Autodesk Inventor part; units mm, degrees
ref_plane "YZ Plane" through (0, 0, 0) normal (1, 0, 0) x (0, 1, 0)
ref_plane "XZ Plane" through (0, 0, 0) normal (0, 1, 0) x (-1, 0, 0)
ref_plane "XY Plane" through (0, 0, 0) normal (0, 0, 1) x (1, 0, 0)
sketch "Sketch1" plane through (0, 0, 0) normal (0, 1, 0) x (-1, 0, 0)
  line L0 (-19.3459, 17.7433) -> (-1.3259, 17.7433)
  line L1 (-1.3259, 0.9433) -> (-19.3459, 0.9433)
  line L2 (-19.3459, 14.5433) -> (-24.3459, 14.5433)
  line L3 (-24.3459, 14.5433) -> (-24.3459, 12.5433)
  line L4 (-24.3459, 12.5433) -> (-19.3459, 12.5433)
  line L5 (-19.3459, 17.7433) -> (-19.3459, 14.5433)
  line L6 (-19.3459, 12.5433) -> (-19.3459, 0.9433)
  line L7 (-1.3259, 17.7433) -> (-1.3259, 14.5433)
  line L8 (-1.3259, 14.5433) -> (3.6741, 14.5433)
  line L9 (3.6741, 14.5433) -> (3.6741, 12.5433)
  line L10 (3.6741, 12.5433) -> (-1.3259, 12.5433)
  line L11 (-1.3259, 12.5433) -> (-1.3259, 0.9433)
  point P0 (0, 0)
  point P1 (-11, -1)
  dimension "d0" = 18.02
  dimension "d1" = 16.8
  dimension "d2" = 2
  dimension "d3" = 5
  dimension "d4" = 3.2
extrude "Extrusion1" add sketch "Sketch1" along normal blind 7.91
properties part number "EMAXES9251"
Read the model definition and answer for the solid it produces. Units are mm, in the model's axes. A direction names the side the tool comes from. Coordinates: 2 decimals unless noted, no trailing zeros. Write each loop counter-clockwise with the first axis right and the second up, starting at its lowest first coordinate (ties: lowest second). Pieces come first, ordered by that corner, then holes. Notation, with made-up numbers: (-17, -36) -> (19, -36) arc R12 ccw to (19, -31) -> close; hole circle Ø4 at (4.25, 46.25). An arc over 180 degrees is marked (long way). Return JSON: item names as keys, results as strings.
(1) Consider line 1 along X through (y, z) = (0.5, 15.5); line 2 along Z through (x, y) = (20.5, 1.25). Determine where each line is inside the solid, lowest interval first. Write a range as from..to.
Answers below:
{"line 1": "1.33..19.35", "line 2": "12.54..14.54"}
(2) Which of the six approach directions +Z, -Z, +X, -X, +Y, -Y give full straight-line access (tool end or side, diameter ignored) to faces 1 (the flat face through (1.326, 4, 7)), 2 (the flat face through (1.326, 4, 16)), 3 (the flat face through (22, 4, 14.543))?
Answers below:
{"face 1": "-Z, -X, +Y, -Y", "face 2": "+Z, -X, +Y, -Y", "face 3": "+Z, +X, +Y, -Y"}
(3) The part is cut by section A-A on y = 2.5. Give the vertices of the cut face in (x, z), then the cut area to 3 significant figures.
Answers below:
{"outline": "(-3.67, 12.54) -> (1.33, 12.54) -> (1.33, 0.94) -> (19.35, 0.94) -> (19.35, 12.54) -> (24.35, 12.54) -> (24.35, 14.54) -> (19.35, 14.54) -> (19.35, 17.74) -> (1.33, 17.74) -> (1.33, 14.54) -> (-3.67, 14.54) -> close", "area": "323 mm^2"}
(4) Each of these flat-tipped pins is pushed along its axis until it touches: P1, Ø2, axis at y = 1.5, z = 7, coming from the +X side; P2, Ø4, axis at y = 2.5, z = 8.5, coming from the -X side; P3, Ø4, axis at x = 22, y = 4.5, coming from the -Z side. Where does it stop, or does it pass through?
Answers below:
{"P1": "x = 19.35", "P2": "x = 1.33", "P3": "z = 12.54"}
(5) The part is cut by section B-B on z = 11.75. Give the vertices of the cut face in (x, y), then the cut area to 3 significant figures.
Answers below:
{"outline": "(1.33, 0) -> (19.35, 0) -> (19.35, 7.91) -> (1.33, 7.91) -> close", "area": "143 mm^2"}
